Read the model definition and answer for the solid it produces. Units are mm, in the model's axes. A direction names the side the tool comes from. Coordinates: 2 decimals unless noted, no trailing zeros. Write each loop counter-clockwise with the first axis right and the second up, starting at its lowest first coordinate (ties: lowest second). Pieces come first, ordered by that corner, then holes. Notation, with made-up numbers: M 27.5,-11 L 48.5,-11 A15 ccw 48.5,6 Z; hole C 23.5,-6 d7. An arc over 180 degrees is marked long. Use a Markdown table: item, result. Add a question column.
from build123d import *

# Parameters (mm, degrees)
F0_R     = 38.1
F0_R_2   = 4.7625
F1_DEPTH = 57.15
F2_SIZE2 = 50.8
F2_SIZE  = 31.75
F4_R     = 19.05
F5_DEPTH = 6.35


with BuildPart() as f1:
    # F0 (on Top) → F1 (new body)
    with BuildSketch(Plane.XY):
        Circle(F0_R)
        Circle(F0_R_2, mode=Mode.SUBTRACT)
    extrude(amount=F1_DEPTH)

    # F2
    f2_edges = [f1.edges().sort_by_distance(p)[0] for p in [
        (-38.1, 0, 57.15),
    ]]
    f2_side = f1.faces().sort_by_distance((-37.022369, 0, 57.15))[0]
    chamfer(f2_edges, length=F2_SIZE, length2=F2_SIZE2, reference=f2_side)

    # F4 (on face) → F5 (cut)
    with BuildSketch(Plane(origin=(0, 0, 0), x_dir=(1, 0, 0), z_dir=(0, 0, -1))):
        Circle(F4_R)
    extrude(amount=-F5_DEPTH, mode=Mode.SUBTRACT)


solid = f1.part
Item 1: Find section A-A on x = 0. Give the vertices of the cut face in (y, z), then the cut area to 3 significant figures.
Item 2: Determine the mould class of faces 1 (the flat face through (4, 4, 6.35)), 2 (the flat face through (1, 5, 57.15)), 3 (the cylindrical face through (-30.235, -23.183, 3.131)) for opening direction Y: pulls with the +Y half, pulls with the -Y half, needs draft (parallel to the pull), parting line crosses it, or undercut.
Item 3: Each of these flat-tipped pins is pushed along its axis until it touches: pin 1 (4 mm diameter, centred on x = -1.5, z = 15, fed in from +Y); pin 2 (12 mm diameter, centred on x = 23.5, z = 11, fed in from +Y); pin 3 (1.5 mm diameter, centred on y = 14, z = 26, fed in from -X). Where does it stop, or does it pass through?
Item 4: Find section D-D on z = 22.5. Give the vertices of the cut face in (x, y) (1 decimal).
Item 5: Find section C-C on z = 38. Give the vertices of the cut face in (x, y) (1 decimal), then the cut area to 3 significant figures.
Item 6: Consider probe 1 along Y at (x, z) = (0, 4.25); probe 2 along X at (y, z) = (0, 39); probe 3 along X at (y, z) = (-17, 5). Determine where each line is inside the solid, lowest interval first.
Item 7: For faces 4 (the cylindrical face through (-15.12, 11.59, 3.13)), 5 (the cylindrical face through (-3.78, -2.9, 31.39)), determine the directions among +Z, -Z, +X, -X, +Y, -Y from which every point of the face is accessible in a straight line to the end or side of a thin tool.
Geometry says:
| question | item | result |
|---|---|---|
| 1 | outline | M -38.1,0 L -19.05,0 L -19.05,6.35 L -4.76,6.35 L -4.76,57.15 L -6.35,57.15 L -38.1,6.35 Z; M 4.76,6.35 L 19.05,6.35 L 19.05,0 L 38.1,0 L 38.1,6.35 L 6.35,57.15 L 4.76,57.15 Z |
| 1 | area | 2,020 mm2 |
| 2 | face 1 | undercut |
| 2 | face 2 | needs draft |
| 2 | face 3 | parting line crosses it |
| 3 | pin 1 | stops at y = 33.91 |
| 3 | pin 2 | stops at y = 32.61 |
| 3 | pin 3 | stops at x = -22.42 |
| 4 | outline | C 0,0 d56; hole C 0,0 d9.5 |
| 5 | outline | C 0,0 d36.6; hole C 0,0 d9.5 |
| 5 | area | 983 mm2 |
| 6 | probe 1 | y = -38.1 to -19.05, 19.05 to 38.1 |
| 6 | probe 2 | x = -17.69 to -4.76, 4.76 to 17.69 |
| 6 | probe 3 | x = -34.1 to -8.6, 8.6 to 34.1 |
| 7 | face 4 | -Z |
| 7 | face 5 | +Z, -Z |
